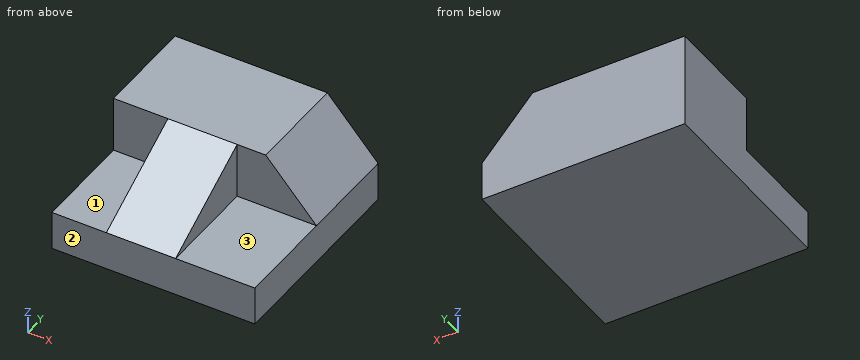
from build123d import *

# Parameters (mm, degrees)
F1_DEPTH = 25.4
F2_W     = 50.8
F2_H     = 9.7338882406
F3_DEPTH = 25.4
F4_W     = 17.3329235986
F4_H     = 14.0222670068
F5_DEPTH = 25.4
F7_DEPTH = 25.4


with BuildPart() as f1:
    # F0 (on Front) → F1 (new body)
    with BuildSketch(Plane.XZ):
        Polygon((0, 23.7561552475), (0, 0), (50.8, 0), (50.8, 9.7338882406), (38.1, 23.7561552475), align=None)
    extrude(amount=F1_DEPTH)

    # F2 (on face) → F3 (join)
    with BuildSketch(Plane.XZ.offset(25.4)):
        with Locations((25.4, 4.8669441203)):
            Rectangle(F2_W, F2_H)
    extrude(amount=F3_DEPTH)

    # F4 (on face) → F5 (join)
    with BuildSketch(Plane.XZ.offset(25.4)):
        with Locations((22.2851852886, 16.7450217441)):
            Rectangle(F4_W, F4_H)
    extrude(amount=F5_DEPTH)

    # F6 (on face) → F7 (cut)
    with BuildSketch(Plane.YZ.offset(30.9516470879)):
        Polygon((-50.8, 23.7561552475), (-50.8, 9.7338882406), (-25.4, 23.7561552475), align=None)
    extrude(amount=-F7_DEPTH, mode=Mode.SUBTRACT)


solid = f1.part
Design review of the part built by this model. Coordinates are the model's own, in mm. Face numbers are marked on the shaded views. A direction names the side the tool comes from. Coordinates: 2 decimals unless noted, no trailing zeros. Write each loop counter-clockwise with the first axis right and the second up, starting at its lowest first coordinate (ties: lowest second). Pieces come first, ordered by that corner, then holes. Notation, with made-up numbers: (60.25, 32.25) -> (90.25, 32.25) arc R15 cw to (90.25, 58.25) -> close; hole circle Ø6 at (48.25, -29.75). An arc over 180 degrees is marked (long way). Write each question's results on one line, items separated by ' | '. Start each with the question number.
(1) Take a section at B-B on z = 20.25. Write out the cut boundary in (x, y), and give its area (3 significant figures).
(2) Take a section at C-C on y = -32. Write out the cut boundary in (x, z), and give its area (3 significant figures).
(3) Take a section at D-D on y = -6. Write out the cut boundary in (x, z), and give its area (3 significant figures).
(4) For line 1 along X through (y, z) = (-32.5, 11); line 2 along Y through (x, z) = (3, 12); line 3 along Z through (x, y) = (16, -35), list the stretches that pass through material, from the lowest coordinate up. Write a range as from..to.
(5) Take a section at A-A on x = 24.5. Write out the cut boundary in (y, z), and give its area (3 significant figures).
(6) Tool access review of the marked faces 1, 2 and 3: name each direction out of +Z, -Z, +X, -X, +Y, -Y from which nothing blocks a thin tool from reaching the whole face with its end or side.
(7) Clearance check with flat-ended pins moving along their axes: P1, Ø3, axis at x = 14, z = 17, coming from the -Y side; P2, Ø8, axis at x = 31.5, z = 18, coming from the -Y side; P3, Ø2, axis at x = 36.5, z = 11.5, coming from the -Y side. State where each tip first meets the part, or that it passes through.
Results found:
1) outline: (0, -25.4) -> (13.62, -25.4) -> (13.62, -31.75) -> (30.95, -31.75) -> (30.95, -25.4) -> (41.28, -25.4) -> (41.28, 0) -> (0, 0) -> close | area: 1,160 mm2
2) outline: (0, 0) -> (50.8, 0) -> (50.8, 9.73) -> (30.95, 9.73) -> (30.95, 20.11) -> (13.62, 20.11) -> (13.62, 9.73) -> (0, 9.73) -> close | area: 674 mm2
3) outline: (0, 0) -> (50.8, 0) -> (50.8, 9.73) -> (38.1, 23.76) -> (0, 23.76) -> close | area: 1,120 mm2
4) line 1: x = 13.62..30.95 | line 2: y = -25.4..0 | line 3: z = 0..18.46
5) outline: (-50.8, 0) -> (0, 0) -> (0, 23.76) -> (-25.4, 23.76) -> (-50.8, 9.73) -> close | area: 1,030 mm2
6) face 1: +Z, -X, -Y | face 2: +Z, -Z, +X, -X, -Y | face 3: +Z, +X, -Y
7) P1: stops at y = -40.36 | P2: stops at y = -43 | P3: stops at y = -25.4
